The model under review builds one solid part; all positions refer to its coordinate system, in mm. A direction names the side the tool comes from. Round coordinates to 2 decimals unless told otherwise and drop trailing zeros. Write each loop counter-clockwise with the first axis right and the second up, starting at its lowest first coordinate (ties: lowest second). Pieces come first, ordered by that corner, then holes. Notation, with made-up numbers: (84.5, 14) - (136.5, 14) arc R15 cw to (136.5, 23) - close; hole circle Ø7 at (29.5, 64.25). An arc over 180 degrees is marked (long way). Use one line per item in the form item = value.
from build123d import *

# Parameters (mm, degrees)
EXTRUDE1_DEPTH                 = 20.6375
EXTRUDE1_DEPTH_BACK            = 20.6375
SKETCH1_R                      = 39.6875
EXTRUDE2_DEPTH                 = 47.625
EXTRUDE2_DEPTH_BACK            = 47.625
SKETCH2_R                      = 15.875
EXTRUDE3_DEPTH                 = 21.43125
EXTRUDE3_DEPTH_BACK            = 21.43125
SKETCH3_R                      = 15.875
EXTRUDE4_DEPTH                 = 44.45
EXTRUDE4_DEPTH_BACK            = 44.45
EXTRUDE5_DEPTH                 = 104.138642279
EXTRUDE5_DEPTH_BACK            = 104.138642279
SKETCH7_R                      = 17.4625
EXTRUDE6_DEPTH                 = 116.854875545
F_9_16_0_5625_DIAMETER_HOLE1_D = 14.2875
F_9_16_0_5625_DIAMETER_HOLE2_D = 14.2875
CHAMFER1_SIZE                  = 1.5875
FILLET1_R                      = 73.66


with BuildPart() as part:
    # Sketch1 → Extrude1 (new, two sides: drawn at the far end of the back side and taken through both)
    with BuildSketch(Plane(origin=(0, 0, 0), x_dir=(0, 0, -1), z_dir=(1, 0, 0)).offset(-EXTRUDE1_DEPTH_BACK)):
        Circle(SKETCH1_R)
    extrude(amount=EXTRUDE1_DEPTH + EXTRUDE1_DEPTH_BACK)



with BuildPart() as body_2:
    # Sketch2 → Extrude2 (new, two sides: drawn at the far end of the back side and taken through both)
    with BuildSketch(Plane.XY.offset(-EXTRUDE2_DEPTH_BACK)):
        with Locations((-33.3375, -55.5625)):
            Circle(SKETCH2_R)
    extrude(amount=EXTRUDE2_DEPTH + EXTRUDE2_DEPTH_BACK)


with BuildPart() as body_3:
    # Sketch3 → Extrude3 (new, two sides: drawn at the far end of the back side and taken through both)
    with BuildSketch(Plane.XY.offset(-EXTRUDE3_DEPTH_BACK)):
        with Locations((-41.275, 55.5625)):
            Circle(SKETCH3_R)
    extrude(amount=EXTRUDE3_DEPTH + EXTRUDE3_DEPTH_BACK)


with BuildPart() as part_1:
    add(part.part)

    add(body_2.part)  # Extrude4 merges body 2

    add(body_3.part)  # Extrude4 merges body 3
    # Sketch4 → Extrude4 (add, two sides: drawn at the far end of the back side and taken through both)
    with BuildSketch(Plane.XY.offset(-EXTRUDE4_DEPTH_BACK)):
        with BuildLine():
            Line((-50.00589462, 42.304027081), (-25.4, 55.5625))
            Line((-25.4, 55.5625), (-3.279393891, 48.933263541))
            Line((-3.279393891, 48.933263541), (-3.279393891, 44.059515259))
            Line((-3.279393891, 44.059515259), (8.797943446, 39.6875))
            Line((8.797943446, 39.6875), (8.797943446, -39.6875))
            Line((8.797943446, -39.6875), (-17.4625, -55.5625))
            Line((-17.4625, -55.5625), (-43.864209099, -43.679570204))
            ThreePointArc((-43.864209099, -43.679570204), (-25.711027758, 0.82823016), (-50.00589462, 42.304027081))
        make_face()
    extrude(amount=EXTRUDE4_DEPTH + EXTRUDE4_DEPTH_BACK)

    # Sketch6 → Extrude5 (cut, two sides: drawn at the far end of the back side and taken through both)
    with BuildSketch(Plane(origin=(0, 0, 0), x_dir=(0, 0, -1), z_dir=(1, 0, 0)).offset(-EXTRUDE5_DEPTH_BACK)):
        with BuildLine():
            Line((-21.43125, 55.5625), (-21.43125, 38.942316616))
            ThreePointArc((-21.43125, 38.942316616), (-38.265007268, 22.618393372), (-44.45, 0))
            Line((-44.45, 0), (-44.45, 55.5625))
            Line((-44.45, 55.5625), (-21.43125, 55.5625))
        make_face()
        with BuildLine():
            Line((21.43125, 55.5625), (21.43125, 38.942316616))
            ThreePointArc((21.43125, 38.942316616), (38.265007268, 22.618393372), (44.45, 0))
            Line((44.45, 0), (44.45, 55.5625))
            Line((44.45, 55.5625), (21.43125, 55.5625))
        make_face()
    extrude(amount=EXTRUDE5_DEPTH + EXTRUDE5_DEPTH_BACK, mode=Mode.SUBTRACT)

    # Sketch7 → Extrude6 (cut, through all)
    with BuildSketch(Plane(origin=(20.6375, 0, 0), x_dir=(0, 0, -1), z_dir=(1, 0, 0))):
        Circle(SKETCH7_R)
    extrude(amount=-EXTRUDE6_DEPTH, mode=Mode.SUBTRACT)

    # 9/16 (0.5625) Diameter Hole1 (through all)
    with Locations(Plane.XY.offset(47.625)):
        with Locations((-33.3375, -55.5625)):
            Hole(F_9_16_0_5625_DIAMETER_HOLE1_D / 2)

    # 9/16 (0.5625) Diameter Hole2 (through all)
    with Locations(Plane.XY.offset(21.43125)):
        with Locations((-41.275, 55.5625)):
            Hole(F_9_16_0_5625_DIAMETER_HOLE2_D / 2)

    # Chamfer1
    chamfer1_edges = [part_1.edges().sort_by_distance(p)[0] for p in [
        (20.6375, 0, 39.6875),
    ]]
    chamfer(chamfer1_edges, length=CHAMFER1_SIZE)

    # Fillet1
    # the kernel refuses this fillet: 73.66 mm, written as the material it takes off along each edge
    with BuildSketch(Plane(origin=(8.797943446, -39.6875, 145.720774821), x_dir=(0, 1, 0), z_dir=(0, 0, -1))) as fillet1_piece_1_section:
        with BuildLine():
            CenterArc((40.508309928, -73.66), FILLET1_R, 90, 49.947360456)
            Line((-15.875, -26.260443446), (0, 0))
            Line((0, 0), (40.508309928, 0))
        make_face()
    fillet1_piece_1 = extrude(amount=145.720774821, mode=Mode.PRIVATE)
    fillet1_piece_1 = fillet1_piece_1 - Plane(origin=(8.797943446, 0, 0), x_dir=(0, 0, -1), z_dir=(-1, 0, 0)) * Cylinder(39.6875, 454, mode=Mode.PRIVATE)
    add(fillet1_piece_1, mode=Mode.SUBTRACT)
    with BuildSketch(Plane(origin=(8.797943446, -39.6875, 0), x_dir=(0, 1, 0), z_dir=(0, 0, -1))) as fillet1_piece_2_section:
        with BuildLine():
            CenterArc((40.508309928, -73.66), FILLET1_R, 90, 49.947360456)
            Line((-15.875, -26.260443446), (0, 0))
            Line((0, 0), (40.508309928, 0))
        make_face()
    fillet1_piece_2 = extrude(amount=145.720774821, mode=Mode.PRIVATE)
    fillet1_piece_2 = fillet1_piece_2 - Plane(origin=(8.797943446, 0, 0), x_dir=(0, 0, -1), z_dir=(-1, 0, 0)) * Cylinder(39.6875, 454, mode=Mode.PRIVATE)
    add(fillet1_piece_2, mode=Mode.SUBTRACT)


solid = part_1.part
(1) Machinability: for faces 1 (the cylindrical face through (-5.062, -42.187, 0.622)), 2 (the cylindrical face through (-48.4, 69.75, -0.3)), 3 (the cylindrical face through (-4.128, 17.314, 2.273)), 4 (the flat face through (8.798, 25, 32)), 5 (the flat face through (-3.279, 47, 0)), which of the approach directions +Z, -Z, +X, -X, +Y, -Y give a long, thin tool a straight path to every point of the face, cutting with its end or side? Answer none if there is none.
Geometry results:
face_1 = +X, -Y
face_2 = +Z, -Z
face_3 = +X, -X
face_4 = +Z, +X, +Y
face_5 = +Z, -Z, +X, +Y
(2) The part is to be moulded in two halves that separate along Y. For faces 6 (the cylindrical face through (-12.674, 22.904, -38.095)), 7 (the cylindrical face through (-36.01, 60.39, -0.3)), 8 (the flat face through (-26.5, -58.9, 47.625)), 9 (the cylindrical face through (7.698, -36.836, -14.771)), say which applies: +Y half, -Y half, draft (parallel to the pull), parting line (faces both ways), or undercut.
Geometry results:
face_6 = +Y half
face_7 = undercut
face_8 = draft
face_9 = parting line
(3) Add section B-B on x = 16.5. Write out the cut boundary in (y, z) (1 decimal), then the cut area to 3 significant figures.
Geometry results:
outline = circle Ø79.4 at (0, 0); hole circle Ø34.9 at (0, 0)
area = 3,990 mm2
(4) To check wall thickness, follow L1, parallel to Z at x = 3.5, y = 0; L2, parallel to Z at x = -46.5, y = 48.5; L3, parallel to Y at x = -44, z = 1.5. State the ranges of each line that lie inside material, in increasing order.
Geometry results:
L1 = -44.45 to -17.46, 17.46 to 44.45
L2 = -21.43 to 21.43
L3 = -67.32 to -43.8, 37.72 to 48.96, 62.17 to 71.2
(5) Add section A-A on y = -50.5. Write out the cut boundary in (x, z) (3 decimals).
Geometry results:
outline = (-48.384, -47.625) - (-38.378, -47.625) - (-38.378, 47.625) - (-48.384, 47.625) - close; (-28.297, -47.625) - (-18.291, -47.625) - (-18.291, -44.45) - (-12.023, -44.45) - (-12.023, 44.45) - (-18.291, 44.45) - (-18.291, 47.625) - (-28.297, 47.625) - close
(6) Insertion check: P1, Ø12, axis at x = 12.5, y = -16.5, coming from the -Z side; P2, Ø12, axis at y = -49, z = 15.5, coming from the +X side; P3, Ø1.5, axis at x = -6.5, z = 26, coming from the -Y side; P4, Ø9.5, axis at x = -12, y = 59.5, coming from the +Z side. Each pin has a flat end and moves straight along its axis. Give the tip position at first contact, or say it passes through.
Geometry results:
P1 = -44.45
P2 = -5.65
P3 = -45.08
P4 = through
